Here's how the part is built. I have some questions about the finished solid (model axes, mm). A direction names the side the tool comes from. Coordinates: 2 decimals unless noted, no trailing zeros. Write each loop counter-clockwise with the first axis right and the second up, starting at its lowest first coordinate (ties: lowest second). Pieces come first, ordered by that corner, then holes.
```python
from build123d import *

# Parameters (mm, degrees)
F0_W     = 115
F0_H     = 210
F0_R     = 20.108519
F1_DEPTH = 1.5


with BuildPart() as f1:
    # F0 (on Top) → F1 (new body)
    with BuildSketch(Plane.XY):
        Rectangle(F0_W, F0_H)
        with BuildLine():
            Line((-51.202005, -98.838247), (-12.797066, -21.618334))
            ThreePointArc((-12.797066, -21.618334), (-11.038136, -22.567162), (-9.209351, -23.373171))
            Line((-9.209351, -23.373171), (-34.33051, -98.838247))
            Line((-34.33051, -98.838247), (-51.202005, -98.838247))
        make_face(mode=Mode.SUBTRACT)
        with BuildLine():
            Line((-21.377223, -98.838247), (-6.066496, -24.378574))
            ThreePointArc((-6.066496, -24.378574), (-4.466784, -24.721754), (-2.848126, -24.960077))
            Line((-2.848126, -24.960077), (-7.67663, -98.838247))
            Line((-7.67663, -98.838247), (-21.377223, -98.838247))
        make_face(mode=Mode.SUBTRACT)
        with BuildLine():
            ThreePointArc((-20.109431, -15.057491), (-18.389989, -17.115068), (-16.461037, -18.977659))
            Line((-16.461037, -18.977659), (-51.202005, -75.210557))
            Line((-51.202005, -75.210557), (-51.207021, -48.053044))
            Line((-51.207021, -48.053044), (-20.109431, -15.057491))
        make_face(mode=Mode.SUBTRACT)
        with BuildLine():
            ThreePointArc((-24.141339, -6.950756), (-23.441886, -9.033009), (-22.563215, -11.046202))
            Line((-22.563215, -11.046202), (-51.210452, -29.471497))
            Line((-51.210452, -29.471497), (-51.213243, -14.361147))
            Line((-51.213243, -14.361147), (-24.141339, -6.950756))
        make_face(mode=Mode.SUBTRACT)
        with BuildLine():
            Line((7.67663, -98.838247), (2.848126, -24.960077))
            ThreePointArc((2.848126, -24.960077), (4.466784, -24.721754), (6.066496, -24.378574))
            Line((6.066496, -24.378574), (21.377223, -98.838247))
            Line((21.377223, -98.838247), (7.67663, -98.838247))
        make_face(mode=Mode.SUBTRACT)
        with BuildLine():
            Line((34.33051, -98.838247), (9.209351, -23.373171))
            ThreePointArc((9.209351, -23.373171), (11.038136, -22.567162), (12.797066, -21.618334))
            Line((12.797066, -21.618334), (51.202005, -98.838247))
            Line((51.202005, -98.838247), (34.33051, -98.838247))
        make_face(mode=Mode.SUBTRACT)
        with BuildLine():
            Line((51.202005, -75.210557), (16.461037, -18.977659))
            ThreePointArc((16.461037, -18.977659), (18.389989, -17.115068), (20.109431, -15.057491))
            Line((20.109431, -15.057491), (51.207021, -48.053044))
            Line((51.207021, -48.053044), (51.202005, -75.210557))
        make_face(mode=Mode.SUBTRACT)
        with BuildLine():
            Line((51.210452, -29.471497), (22.563215, -11.046202))
            ThreePointArc((22.563215, -11.046202), (23.441886, -9.033009), (24.141339, -6.950756))
            Line((24.141339, -6.950756), (51.213243, -14.361147))
            Line((51.213243, -14.361147), (51.210452, -29.471497))
        make_face(mode=Mode.SUBTRACT)
        with BuildLine():
            ThreePointArc((-24.952535, 2.91346), (-25.122047, 0), (-24.952535, -2.91346))
            Line((-24.952535, -2.91346), (-51.213243, -5.612732))
            Line((-51.213243, -5.612732), (-51.213243, 5.612732))
            Line((-51.213243, 5.612732), (-24.952535, 2.91346))
        make_face(mode=Mode.SUBTRACT)
        with BuildLine():
            Line((-51.210452, 29.471497), (-22.563215, 11.046202))
            ThreePointArc((-22.563215, 11.046202), (-23.441886, 9.033009), (-24.141339, 6.950756))
            Line((-24.141339, 6.950756), (-51.213243, 14.361147))
            Line((-51.213243, 14.361147), (-51.210452, 29.471497))
        make_face(mode=Mode.SUBTRACT)
        with BuildLine():
            Line((-51.202005, 75.210557), (-16.461037, 18.977659))
            ThreePointArc((-16.461037, 18.977659), (-18.389989, 17.115068), (-20.109431, 15.057491))
            Line((-20.109431, 15.057491), (-51.207021, 48.053044))
            Line((-51.207021, 48.053044), (-51.202005, 75.210557))
        make_face(mode=Mode.SUBTRACT)
        with BuildLine():
            Line((-34.33051, 98.838247), (-9.209351, 23.373171))
            ThreePointArc((-9.209351, 23.373171), (-11.038136, 22.567162), (-12.797066, 21.618334))
            Line((-12.797066, 21.618334), (-51.202005, 98.838247))
            Line((-51.202005, 98.838247), (-34.33051, 98.838247))
        make_face(mode=Mode.SUBTRACT)
        with BuildLine():
            Line((-7.67663, 98.838247), (-2.848126, 24.960077))
            ThreePointArc((-2.848126, 24.960077), (-4.466784, 24.721754), (-6.066496, 24.378574))
            Line((-6.066496, 24.378574), (-21.377223, 98.838247))
            Line((-21.377223, 98.838247), (-7.67663, 98.838247))
        make_face(mode=Mode.SUBTRACT)
        Circle(F0_R, mode=Mode.SUBTRACT)
        with BuildLine():
            ThreePointArc((24.952535, -2.91346), (25.122047, 0), (24.952535, 2.91346))
            Line((24.952535, 2.91346), (51.213243, 5.612732))
            Line((51.213243, 5.612732), (51.213243, -5.612732))
            Line((51.213243, -5.612732), (24.952535, -2.91346))
        make_face(mode=Mode.SUBTRACT)
        with BuildLine():
            ThreePointArc((24.141339, 6.950756), (23.441886, 9.033009), (22.563215, 11.046202))
            Line((22.563215, 11.046202), (51.210452, 29.471497))
            Line((51.210452, 29.471497), (51.213243, 14.361147))
            Line((51.213243, 14.361147), (24.141339, 6.950756))
        make_face(mode=Mode.SUBTRACT)
        with BuildLine():
            ThreePointArc((20.109431, 15.057491), (18.389989, 17.115068), (16.461037, 18.977659))
            Line((16.461037, 18.977659), (51.202005, 75.210557))
            Line((51.202005, 75.210557), (51.207021, 48.053044))
            Line((51.207021, 48.053044), (20.109431, 15.057491))
        make_face(mode=Mode.SUBTRACT)
        with BuildLine():
            ThreePointArc((6.066496, 24.378574), (4.466784, 24.721754), (2.848126, 24.960077))
            Line((2.848126, 24.960077), (7.67663, 98.838247))
            Line((7.67663, 98.838247), (21.377223, 98.838247))
            Line((21.377223, 98.838247), (6.066496, 24.378574))
        make_face(mode=Mode.SUBTRACT)
        with BuildLine():
            ThreePointArc((12.797066, 21.618334), (11.038136, 22.567162), (9.209351, 23.373171))
            Line((9.209351, 23.373171), (34.33051, 98.838247))
            Line((34.33051, 98.838247), (51.202005, 98.838247))
            Line((51.202005, 98.838247), (12.797066, 21.618334))
        make_face(mode=Mode.SUBTRACT)
    extrude(amount=F1_DEPTH)


solid = f1.part
```
1) I need wall thicknesses on probe 1 along Y at (x, z) = (0, 0.5); probe 2 along X at (y, z) = (84, 1.4); probe 3 along X at (y, z) = (6.5, 0.7). Which ranges of each line are inside material? Lowest first, please.
Values follow:
probe 1: y = -105 to -20.11, 20.11 to 105
probe 2: x = -57.5 to -43.82, -29.39 to -18.33, -6.71 to 6.71, 18.33 to 29.39, 43.82 to 57.5
probe 3: x = -57.5 to -19.03, 19.03 to 57.5
2) Imagine slicing it at B-B on x = 0. Please give me the cut outline in (y, z).
Values follow:
outline: (-105, 0) - (-20.11, 0) - (-20.11, 1.5) - (-105, 1.5) - close; (20.11, 0) - (105, 0) - (105, 1.5) - (20.11, 1.5) - close
3) We'd pull the mould along Y, two halves only. Please class faces 3 (the face through (-14, -22, 0)), 4 (the face through (-34.075, 47.488, 0.74)): pulls with the +Y half, pulls with the -Y half, needs draft (parallel to the pull), parting line crosses it, or undercut.
Values follow:
face 3: needs draft
face 4: undercut
4) Imagine slicing it at D-D on y = 44.5. Please give me the cut outline in (x, z), then the cut area to 3 significant figures.
Values follow:
outline: (-57.5, 0) - (-47.86, 0) - (-47.86, 1.5) - (-57.5, 1.5) - close; (-32.23, 0) - (-24.18, 0) - (-24.18, 1.5) - (-32.23, 1.5) - close; (-16.24, 0) - (-10.2, 0) - (-10.2, 1.5) - (-16.24, 1.5) - close; (-4.13, 0) - (4.13, 0) - (4.13, 1.5) - (-4.13, 1.5) - close; (10.2, 0) - (16.24, 0) - (16.24, 1.5) - (10.2, 1.5) - close; (24.18, 0) - (32.23, 0) - (32.23, 1.5) - (24.18, 1.5) - close; (47.86, 0) - (57.5, 0) - (57.5, 1.5) - (47.86, 1.5) - close
area: 83.6 mm2
5) On a 3-axis mill with a long thin cutter (end or side, diameter ignored), from which of +Z, -Z, +X, -X, +Y, -Y can I reach the whole of each face in a straight line? I mean faces 1 (the face through (-35.441, 31.324, 0.74)), 2 (the face through (-14, -22, 1.5)). Say none if no direction works.
Values follow:
face 1: +Z, -Z
face 2: +Z, +X, -X, +Y, -Y
6) Imagine slicing it at C-C on z = 0.55. Count the separate pieces of the cut face and the enclosed holes in it, then the cut area to 3 significant figures.
Values follow:
separate pieces: 1
enclosed holes: 19
area: 13,200 mm2
7) Imagine slicing it at A-A on y = 0. Please give me the cut outline in (x, z).
Values follow:
outline: (-57.5, 0) - (-51.21, 0) - (-51.21, 1.5) - (-57.5, 1.5) - close; (-25.12, 0) - (-20.11, 0) - (-20.11, 1.5) - (-25.12, 1.5) - close; (20.11, 0) - (25.12, 0) - (25.12, 1.5) - (20.11, 1.5) - close; (51.21, 0) - (57.5, 0) - (57.5, 1.5) - (51.21, 1.5) - close
8) Will these pins go through, and if not, where does the flat tip stop? pin 1 (12 mm diameter, centred on x = -45, y = 39.5, fed in from -Z); pin 2 (6 mm diameter, centred on x = 38, y = 47.5, fed in from -Z).
Values follow:
pin 1: stops at z = 0
pin 2: passes through
